from build123d import *

# Parameters (mm, degrees)
SKETCH_1_R          = 71
SKETCH_1_R_2        = 1.25
SKETCH_1_R_3        = 7.5
EXTRUDE_1_DEPTH     = 3
CUT_EXTRUDE_1_REACH = 102.454
SKETCH_2_R          = 2.5
CUT_EXTRUDE_2_REACH = 102.454
CUT_EXTRUDE_3_REACH = 102.454
SKETCH_4_R          = 7.5
FILLET_1_R          = 5


with BuildPart() as part:
    # 草图1 → 凸台-拉伸1 (new body)
    with BuildSketch(Plane.XY):
        Circle(SKETCH_1_R)
        with Locations((0, 65)):
            Circle(SKETCH_1_R_2, mode=Mode.SUBTRACT)
        with Locations((56.291651246, 32.5)):
            Circle(SKETCH_1_R_2, mode=Mode.SUBTRACT)
        with Locations((56.291651246, -32.5)):
            Circle(SKETCH_1_R_2, mode=Mode.SUBTRACT)
        with Locations((0, -65)):
            Circle(SKETCH_1_R_2, mode=Mode.SUBTRACT)
        with Locations((-56.291651246, -32.5)):
            Circle(SKETCH_1_R_2, mode=Mode.SUBTRACT)
        with Locations((-56.291651246, 32.5)):
            Circle(SKETCH_1_R_2, mode=Mode.SUBTRACT)
        with Locations((-29.074072829, 32.680101792)):
            Circle(SKETCH_1_R_2, mode=Mode.SUBTRACT)
        with Locations((-13.764761936, 41.518936557)):
            Circle(SKETCH_1_R_2, mode=Mode.SUBTRACT)
        with Locations((-4.925927171, 26.209625665)):
            Circle(SKETCH_1_R_2, mode=Mode.SUBTRACT)
        with Locations((-20.235238064, 17.3707909)):
            Circle(SKETCH_1_R_2, mode=Mode.SUBTRACT)
        with Locations(Location((29.074072829, -32.680101792, 0), (0, 0, 180))):
            Circle(SKETCH_1_R_2, mode=Mode.SUBTRACT)
        with Locations(Location((20.235238064, -17.3707909, 0), (0, 0, 180))):
            Circle(SKETCH_1_R_2, mode=Mode.SUBTRACT)
        with Locations(Location((4.925927171, -26.209625665, 0), (0, 0, 180))):
            Circle(SKETCH_1_R_2, mode=Mode.SUBTRACT)
        with Locations(Location((13.764761936, -41.518936557, 0), (0, 0, 180))):
            Circle(SKETCH_1_R_2, mode=Mode.SUBTRACT)
        with Locations((-17, 29.444863729)):
            Circle(SKETCH_1_R_3, mode=Mode.SUBTRACT)
        with Locations(Location((17, -29.444863729, 0), (0, 0, 180))):
            Circle(SKETCH_1_R_3, mode=Mode.SUBTRACT)
        with Locations((32.5, 56.291651246)):
            Circle(SKETCH_1_R_2, mode=Mode.SUBTRACT)
        with Locations((-32.5, 56.291651246)):
            Circle(SKETCH_1_R_2, mode=Mode.SUBTRACT)
        with Locations((-65, 0)):
            Circle(SKETCH_1_R_2, mode=Mode.SUBTRACT)
        with Locations((-32.5, -56.291651246)):
            Circle(SKETCH_1_R_2, mode=Mode.SUBTRACT)
        with Locations((32.5, -56.291651246)):
            Circle(SKETCH_1_R_2, mode=Mode.SUBTRACT)
        with Locations((65, 0)):
            Circle(SKETCH_1_R_2, mode=Mode.SUBTRACT)
    extrude(amount=EXTRUDE_1_DEPTH)

    # 草图2 → 切除-拉伸1 (cut, up to next)
    with BuildSketch(Plane.XY.offset(3), mode=Mode.PRIVATE) as cut_extrude_1_sk1:
        with Locations((-48.260799916, 40.49561941)):
            Circle(SKETCH_2_R)
    cut_extrude_1_tool1 = extrude(cut_extrude_1_sk1.sketch, amount=-CUT_EXTRUDE_1_REACH, mode=Mode.PRIVATE) & part.part
    add(cut_extrude_1_tool1.solids().sort_by_distance((-48.2608, 40.495619, 3))[0], mode=Mode.SUBTRACT)

    # 草图3 → 切除-拉伸2 (cut, up to next)
    with BuildSketch(Plane.XY.offset(3), mode=Mode.PRIVATE) as cut_extrude_2_sk1:
        with BuildLine():
            Line((-43.473901737, 35.299006612), (-19.820508076, -5.669872981))
            Line((-19.820508076, -5.669872981), (-50.803726564, -23.558042516))
            ThreePointArc((-50.803726564, -23.558042516), (-55.570728424, 6.920559405), (-43.473901737, 35.299006612))
        make_face()
    cut_extrude_2_tool1 = extrude(cut_extrude_2_sk1.sketch, amount=-CUT_EXTRUDE_2_REACH, mode=Mode.PRIVATE) & part.part
    # 草图3 → 切除-拉伸2 (cut, up to next)
    with BuildSketch(Plane.XY.offset(3), mode=Mode.PRIVATE) as cut_extrude_2_sk2:
        with BuildLine():
            Line((-8.832885586, 55.299006612), (14.820508076, 14.330127019))
            Line((14.820508076, 14.330127019), (45.803726564, 32.218296554))
            ThreePointArc((45.803726564, 32.218296554), (21.791983959, 51.585942224), (-8.832885586, 55.299006612))
        make_face()
    cut_extrude_2_tool2 = extrude(cut_extrude_2_sk2.sketch, amount=-CUT_EXTRUDE_2_REACH, mode=Mode.PRIVATE) & part.part
    # 草图3 → 切除-拉伸2 (cut, up to next)
    with BuildSketch(Plane.XY.offset(3), mode=Mode.PRIVATE) as cut_extrude_2_sk3:
        with BuildLine():
            Line((19.820508076, 5.669872981), (50.803726564, 23.558042516))
            ThreePointArc((50.803726564, 23.558042516), (55.570728424, -6.920559405), (43.473901737, -35.299006612))
            Line((43.473901737, -35.299006612), (19.820508076, 5.669872981))
        make_face()
    cut_extrude_2_tool3 = extrude(cut_extrude_2_sk3.sketch, amount=-CUT_EXTRUDE_2_REACH, mode=Mode.PRIVATE) & part.part
    # 草图3 → 切除-拉伸2 (cut, up to next)
    with BuildSketch(Plane.XY.offset(3), mode=Mode.PRIVATE) as cut_extrude_2_sk4:
        with BuildLine():
            Line((-14.820508076, -14.330127019), (-45.803726564, -32.218296554))
            ThreePointArc((-45.803726564, -32.218296554), (-21.791983959, -51.585942224), (8.832885586, -55.299006612))
            Line((8.832885586, -55.299006612), (-14.820508076, -14.330127019))
        make_face()
    cut_extrude_2_tool4 = extrude(cut_extrude_2_sk4.sketch, amount=-CUT_EXTRUDE_2_REACH, mode=Mode.PRIVATE) & part.part
    add(cut_extrude_2_tool1.solids().sort_by_distance((-41.626791, 3.251163, 3))[0], mode=Mode.SUBTRACT)
    add(cut_extrude_2_tool2.solids().sort_by_distance((17.997806, 37.67544, 3))[0], mode=Mode.SUBTRACT)
    add(cut_extrude_2_tool3.solids().sort_by_distance((41.626791, -3.251163, 3))[0], mode=Mode.SUBTRACT)
    add(cut_extrude_2_tool4.solids().sort_by_distance((-17.997806, -37.67544, 3))[0], mode=Mode.SUBTRACT)

    # 草图4 → 切除-拉伸3 (cut, up to next)
    with BuildSketch(Plane.XY.offset(3), mode=Mode.PRIVATE) as cut_extrude_3_sk1:
        Circle(SKETCH_4_R)
    cut_extrude_3_tool1 = extrude(cut_extrude_3_sk1.sketch, amount=-CUT_EXTRUDE_3_REACH, mode=Mode.PRIVATE) & part.part
    add(cut_extrude_3_tool1.solids().sort_by_distance((0, 0, 3))[0], mode=Mode.SUBTRACT)

    # 圆角1
    fillet_1_edges = [part.edges().sort_by_distance(p)[0] for p in [
        (8.832885586, -55.299006612, 1.5),
        (-45.803726564, -32.218296554, 1.5),
        (-14.820508076, -14.330127019, 1.5),
        (-8.832885586, 55.299006612, 1.5),
        (45.803726564, 32.218296554, 1.5),
        (14.820508076, 14.330127019, 1.5),
        (50.803726564, 23.558042516, 1.5),
        (43.473901737, -35.299006612, 1.5),
        (19.820508076, 5.669872981, 1.5),
        (-50.803726564, -23.558042516, 1.5),
        (-43.473901737, 35.299006612, 1.5),
        (-19.820508076, -5.669872981, 1.5),
    ]]
    fillet(fillet_1_edges, radius=FILLET_1_R)


solid = part.part
CAD build for the part. Positions are in the model's coordinates, mm. A direction names the side the tool comes from. Round coordinates to 2 decimals unless told otherwise and drop trailing zeros. Write each loop counter-clockwise with the first axis right and the second up, starting at its lowest first coordinate (ties: lowest second). Pieces come first, ordered by that corner, then holes. Notation, with made-up numbers: M -11.5,54.25 L 33.5,54.25 A15 ccw 33.5,60.25 Z; hole C 67,12 d7. An arc over 180 degrees is marked long. Put each result on its own line as item: value. Start each with the question number.
1) Saw through at B-B, the plane z = 1.1. Count the separate pieces of the cut face and the enclosed holes in it, and give its area (3 significant figures).
2) Pull direction X, two halves, no side cores. Call faces 3 (the flat face through (-31.054, 13.787, 1.521)), 4 (the cylindrical face through (-15.39, -69.31, 1.48)), 5 (the flat face through (-1, -15, 3)): pulls with the +X half, pulls with the -X half, needs draft (parallel to the pull), parting line crosses it, or undercut.
3) Saw through at A-A, the plane x = 17. Write the cut outline in (y, z).
4) Drill centre lines: probe 1 along Y at (x, z) = (-46, 0.8); probe 2 along X at (y, z) = (-29.5, 1.8); probe 3 along Y at (x, z) = (27.5, 0.85). Where is each one in solid material? Low to high. Write a range as [from, to].
5) 3-axis set-ups, long thin cutter, end or side, ignore diameter. For faces 1 (the cylindrical face through (-23.11, -51.01, 1.52)), 2 (the flat face through (-1, -15, 0)): which of +Z, -Z, +X, -X, +Y, -Y reach the whole face in a straight line?
6) Pin check, flat tip, straight feed: pin 1 Ø1.5 at (x, y) = (0, 65) entering from -Z. Stop position of the tip, or through.
Resolved:
1. separate pieces: 1
1. enclosed holes: 28
1. area: 10,600 mm²
2. face 3: undercut
2. face 4: parting line crosses it
2. face 5: needs draft
3. outline: M -68.93,0 L -36.94,0 L -36.94,3 L -68.93,3 Z; M -21.94,0 L 16.17,0 L 16.17,3 L -21.94,3 Z; M 53.36,0 L 68.93,0 L 68.93,3 L 53.36,3 Z
4. probe 1: [-54.08, -20.78], [30.52, 39.43], [41.56, 54.08]
4. probe 2: [-64.58, -41.08], [-6.06, 9.5], [24.5, 40.31], [47.44, 64.58]
4. probe 3: [-65.46, -7.63], [10.1, 21.65], [48.78, 65.46]
5. face 1: +Z, -Z
5. face 2: -Z, +X, -X, +Y, -Y
6. pin 1: through
